from build123d import *

# Parameters (mm, degrees)
F1_DEPTH = 10
F2_R     = 20
F3_DEPTH = 20
F4_R     = 10
F5_DEPTH = 58.8
F6_W     = 50
F6_H     = 12
F7_DEPTH = 6
F9_DEPTH = 10


with BuildPart() as f1:
    # F0 (on Top) → F1 (new body)
    with BuildSketch(Plane.XY):
        with BuildLine():
            Line((45.792472, 20), (0, 20))
            ThreePointArc((0, 20), (-20, 0), (0, -20))
            Line((0, -20), (45.792472, -20))
            ThreePointArc((45.792472, -20), (65.792472, 0), (45.792472, 20))
        make_face()
    extrude(amount=F1_DEPTH)

    # F2 (on face) → F3 (join)
    with BuildSketch(Plane.XY.offset(10)):
        Circle(F2_R)
    extrude(amount=F3_DEPTH)

    # F4 (on face) → F5 (cut)
    with BuildSketch(Plane.XY.offset(30)):
        Circle(F4_R)
    extrude(amount=-F5_DEPTH, mode=Mode.SUBTRACT)

    # F6 (on face) → F7 (cut)
    with BuildSketch(Plane.XY.offset(30)):
        Rectangle(F6_W, F6_H)
    extrude(amount=-F7_DEPTH, mode=Mode.SUBTRACT)

    # F8 (on face) → F9 (cut)
    with BuildSketch(Plane.XY.offset(10)):
        with BuildLine():
            Line((45.792472, 7.5), (30.792472, 7.5))
            ThreePointArc((30.792472, 7.5), (23.292472, 0), (30.792472, -7.5))
            Line((30.792472, -7.5), (45.792472, -7.5))
            ThreePointArc((45.792472, -7.5), (53.292472, 0), (45.792472, 7.5))
        make_face()
    extrude(amount=-F9_DEPTH, mode=Mode.SUBTRACT)


solid = f1.part
Can you work these out from the model? Positions are in its coordinate system, mm. A direction names the side the tool comes from. Coordinates: 2 decimals unless noted, no trailing zeros. Write each loop counter-clockwise with the first axis right and the second up, starting at its lowest first coordinate (ties: lowest second). Pieces come first, ordered by that corner, then holes. Notation, with made-up numbers: (79, 2.25) -> (95, 2.25) arc R8 cw to (95, 17.25) -> close; hole circle Ø11 at (-32.5, 2.5). An arc over 180 degrees is marked (long way). Write each question's results on one line, items separated by ' | '. Start each with the question number.
Item 1: If we section it at C-C, the plane x = -2: Write out the boundary of the cut face in (y, z).
Item 2: On a 3-axis mill with a long thin cutter (end or side, diameter ignored), from which of +Z, -Z, +X, -X, +Y, -Y can I reach the whole of each face in a straight line? I mean faces 1 (the cylindrical face through (-19.98, 0.88, 14.79)), 2 (the flat face through (13, -6, 27)), 3 (the flat face through (38, -7.5, 5)), 4 (the flat face through (0, 13, 30)). Say none if no direction works.
Item 3: Please list where these lines run through material, in increasing order: probe 1 along X at (y, z) = (0, 8); probe 2 along X at (y, z) = (0, 18).
Item 4: I'm going to push flat-ended pins straight in: P1, Ø1, axis at x = 27.5, y = -11, coming from the -Z side; P2, Ø3, axis at x = -11, z = 27, coming from the +Y side; P3, Ø5, axis at x = 14, z = 26.5, coming from the +Y side; P4, Ø1.8, axis at x = -15.5, z = 27.5, coming from the -Y side. Where does each tip first touch, or does it pass through?
Item 5: If we section it at A-A, the plane z = 27: Write out the boundary of the cut face in (x, y).
Item 6: Thinking about a two-plate mould opening in Y: for faces 5 (the cylindrical face through (65.788, -0.44, 4.93)), 6 (the flat face through (-14, 0, 24)), 7 (the flat face through (0, -13, 30)), which applies, released by +Y, released by -Y, zero draft, split by the parting line, or undercut?
Item 7: If we section it at B-B, the plane y = 0: Write out the boundary of the cut face in (x, z), and give its area (3 significant figures).
Item 8: If we section it at D-D, the plane x = -12: Write out the boundary of the cut face in (y, z).
Answer block:
1) outline: (-19.9, 0) -> (-9.8, 0) -> (-9.8, 30) -> (-19.9, 30) -> close; (9.8, 0) -> (19.9, 0) -> (19.9, 30) -> (9.8, 30) -> close
2) face 1: +Z | face 2: +Z, +X, -X | face 3: +Z, -Z | face 4: +Z, +X, -X, +Y, -Y
3) probe 1: -20 to -10, 10 to 23.29, 53.29 to 65.79 | probe 2: -20 to -10, 10 to 20
4) P1: z = 0 | P2: y = 17.6 | P3: y = 16.36 | P4: y = -13.67
5) outline: (-19.08, -6) arc R20 ccw to (19.08, -6) -> (8, -6) arc R10 cw to (-8, -6) -> close; (-19.08, 6) -> (-8, 6) arc R10 cw to (8, 6) -> (19.08, 6) arc R20 ccw to start
6) face 5: split by the parting line | face 6: undercut | face 7: zero draft
7) outline: (-20, 0) -> (-10, 0) -> (-10, 24) -> (-20, 24) -> close; (10, 0) -> (23.29, 0) -> (23.29, 10) -> (20, 10) -> (20, 24) -> (10, 24) -> close; (53.29, 0) -> (65.79, 0) -> (65.79, 10) -> (53.29, 10) -> close | area: 638 mm²
8) outline: (-16, 0) -> (16, 0) -> (16, 30) -> (6, 30) -> (6, 24) -> (-6, 24) -> (-6, 30) -> (-16, 30) -> close
